Here's the drawing with two shaded views (mm, measured from the low corner). I have some questions. A direction names the side the tool comes from. Coordinates: 2 decimals unless noted, no trailing zeros. Loops run counter-clockwise (first coordinate to the right, second up) from the corner with the lowest first, then second, coordinate; pieces in that order, holes last. Notation, with made-up numbers: (-11.5, 33) - (27.5, 33) arc R22 cw to (27.5, 67) - close; hole circle Ø9 at (84, 57.25). An arc over 180 degrees is marked (long way). Use a Markdown table: item, result.
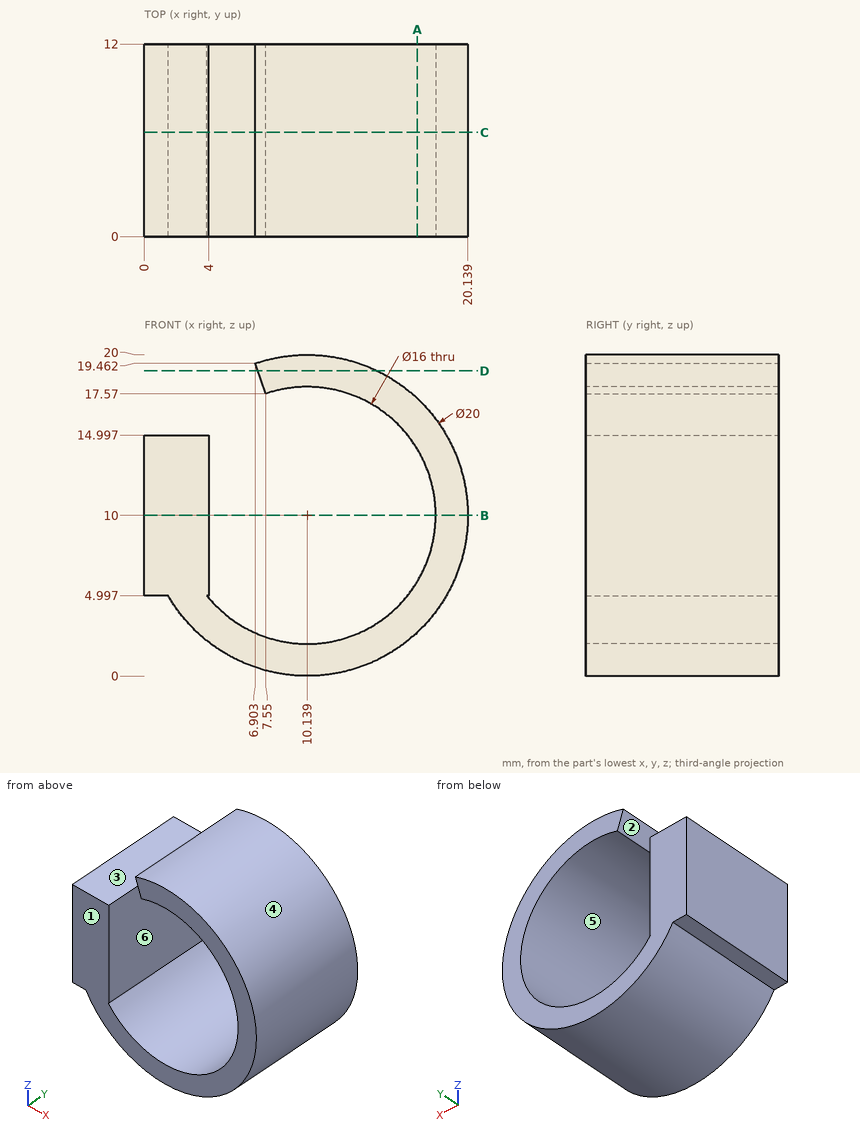
Q1. Will these pins go through, and if not, where does the flat tip stop? P1, Ø3, axis at y = 2.5, z = 15.5, coming from the +X side (1 decimal); P2, Ø3, axis at x = 2.5, y = 6.5, coming from the +Z side; P3, Ø1, axis at y = 7.5, z = 15, coming from the +X side.
Check values:
| item | result |
|---|---|
| P1 | x = 19.3 |
| P2 | z = 15 |
| P3 | x = 19.07 |
Q2. I want a section at A-A, the plane x = 17. Write out the boundary of the cut face in (y, z) (1 decimal).
Check values:
| item | result |
|---|---|
| outline | (0, 2.7) - (12, 2.7) - (12, 5.9) - (0, 5.9) - close; (0, 14.1) - (12, 14.1) - (12, 17.3) - (0, 17.3) - close |
Q3. I want a section at C-C, the plane y = 6.5. Write out the boundary of the cut face in (x, z).
Check values:
| item | result |
|---|---|
| outline | (0, 5) - (1.48, 5) arc R10 ccw (long way) to (6.9, 19.46) - (7.55, 17.57) arc R8 cw (long way) to (3.9, 5) - (4, 5) - (4, 15) - (0, 15) - close |
Q4. Which directions (+Z, -Z, +X, -X, +Y, -Y) give clear straight access to the entire face, cutting with the end or side of a thin tool? Please do the marked faces 1 and 2.
Check values:
| item | result |
|---|---|
| face 1 | +Z, -Z, +X, -X, -Y |
| face 2 | -X, +Y, -Y |
Q5. I want a section at B-B, the plane z = 10. Write out the boundary of the cut face in (x, y), then the cut area to 3 significant figures.
Check values:
| item | result |
|---|---|
| outline | (0, 0) - (4, 0) - (4, 12) - (0, 12) - close; (18.14, 0) - (20.14, 0) - (20.14, 12) - (18.14, 12) - close |
| area | 72.0 mm^2 |
Q6. If we mould it in two halves opening along X, with no side actions, what happens to the marked faces 3, 4, 5 and 6? For each: pulls with the +X half, pulls with the -X half, needs draft (parallel to the pull), parting line crosses it, or undercut.
Check values:
| item | result |
|---|---|
| face 3 | needs draft |
| face 4 | parting line crosses it |
| face 5 | undercut |
| face 6 | undercut |
Q7. Please list where these lines run through material, in increasing order: L1, parallel to X at y = 5.5, z = 10; L2, parallel to Z at x = 11.25, y = 8.5; L3, parallel to X at y = 6, z = 12 (1 decimal). Write a range as from..to.
Check values:
| item | result |
|---|---|
| L1 | 0..4, 18.14..20.14 |
| L2 | 0.06..2.08, 17.92..19.94 |
| L3 | 0..4, 17.9..19.9 |
Q8. I want a section at D-D, the plane z = 19. Write out the boundary of the cut face in (x, y).
Check values:
| item | result |
|---|---|
| outline | (7.06, 0) - (14.5, 0) - (14.5, 12) - (7.06, 12) - close |
